from build123d import *

# Parameters (mm, degrees)
SKETCH_1_R          = 30
EXTRUDE_1_DEPTH     = 10
SKETCH_2_R          = 7.5
CUT_EXTRUDE_1_DEPTH = 44.588989435
SKETCH_3_R          = 2
CUT_EXTRUDE_2_DEPTH = 44.588989435


with BuildPart() as part:
    # 草图1 → 凸台-拉伸1 (new body)
    with BuildSketch(Plane.XY):
        Circle(SKETCH_1_R)
    extrude(amount=EXTRUDE_1_DEPTH)

    # 草图2 → 切除-拉伸1 (cut, through all)
    with BuildSketch(Plane.XY):
        Circle(SKETCH_2_R)
    extrude(amount=CUT_EXTRUDE_1_DEPTH, mode=Mode.SUBTRACT)

    # 草图3 → 切除-拉伸2 (cut, through all)
    with BuildSketch(Plane.XY):
        with Locations((24, 0)):
            Circle(SKETCH_3_R)
        with Locations((20.78461, 12)):
            Circle(SKETCH_3_R)
        with Locations((12, 20.78461)):
            Circle(SKETCH_3_R)
        with Locations((0, 24)):
            Circle(SKETCH_3_R)
        with Locations((-12, 20.78461)):
            Circle(SKETCH_3_R)
        with Locations((-20.78461, 12)):
            Circle(SKETCH_3_R)
        with Locations((-24, 0)):
            Circle(SKETCH_3_R)
        with Locations((-20.78461, -12)):
            Circle(SKETCH_3_R)
        with Locations((-12, -20.78461)):
            Circle(SKETCH_3_R)
        with Locations((0, -24)):
            Circle(SKETCH_3_R)
        with Locations((12, -20.78461)):
            Circle(SKETCH_3_R)
        with Locations((20.78461, -12)):
            Circle(SKETCH_3_R)
    extrude(amount=CUT_EXTRUDE_2_DEPTH, mode=Mode.SUBTRACT)


solid = part.part
Can you work these out from the model? Positions are in its coordinate system, mm. Round coordinates to 2 decimals unless told otherwise and drop trailing zeros. Loops run counter-clockwise (first coordinate to the right, second up) from the corner with the lowest first, then second, coordinate; pieces in that order, holes last. Notation, with made-up numbers: (74.5, 2.5) - (115.5, 2.5) arc R37 cw to (115.5, 41.5) - close; hole circle Ø1 at (74.25, 40). An arc over 180 degrees is marked (long way). Use CSV: the item, a comma, the result in double quotes. Start each with the question number.
1) Please list where these lines run through material, in increasing order: probe 1 along X at (y, z) = (13, 1); probe 2 along Y at (x, z) = (12, 7.75); probe 3 along Y at (x, z) = (-21, 1.5). Write a range as [from, to].
2) If we section it at B-B on y = -12: Write out the boundary of the cut face in (x, z), plus the area to 3 significant figures.
3) For pin 1 Ø1 at (x, z) = (4.5, 8.5) entering from -Y; pin 2 Ø1.5 at (y, z) = (-18, 8) entering from +X; pin 3 Ø1 at (y, z) = (18, 7) entering from -X, each with a flat end and sliding along its axis, tell me the tip position at first contact or that it passes through.
4) If we section it at A-A on x = -24: Write out the boundary of the cut face in (y, z).
5) If we section it at C-C on z = 3.5: Count the separate pieces of the cut face and the enclosed holes in it, plus the area to 3 significant figures.
6) We'd pull the mould along X, two halves only. Please class faces 1 (the cylindrical face through (-26, 0, 5)), 2 (the cylindrical face through (-29.97, 1.32, 4.93)), 3 (the flat face through (6, -6, 0)): released by +X, released by -X, zero draft, split by the parting line, or undercut.
Geometry results:
1,probe 1,"x = [-27.04, -22.52], [-19.05, 19.05], [22.52, 27.04]"
1,probe 2,"y = [-27.5, -22.78], [-18.78, 18.78], [22.78, 27.5]"
1,probe 3,"y = [-21.42, -13.99], [-10.01, 10.01], [13.99, 21.42]"
2,outline,"(-27.5, 0) - (-22.78, 0) - (-22.78, 10) - (-27.5, 10) - close; (-18.78, 0) - (18.78, 0) - (18.78, 10) - (-18.78, 10) - close; (22.78, 0) - (27.5, 0) - (27.5, 10) - (22.78, 10) - close"
2,area,"470 mm2"
3,pin 1,"stops at y = -29.73"
3,pin 2,"stops at x = 24.54"
3,pin 3,"stops at x = -24.37"
4,outline,"(-18, 0) - (-2, 0) - (-2, 10) - (-18, 10) - close; (2, 0) - (18, 0) - (18, 10) - (2, 10) - close"
5,separate pieces,"1"
5,enclosed holes,"13"
5,area,"2,500 mm2"
6,face 1,"undercut"
6,face 2,"split by the parting line"
6,face 3,"zero draft"
